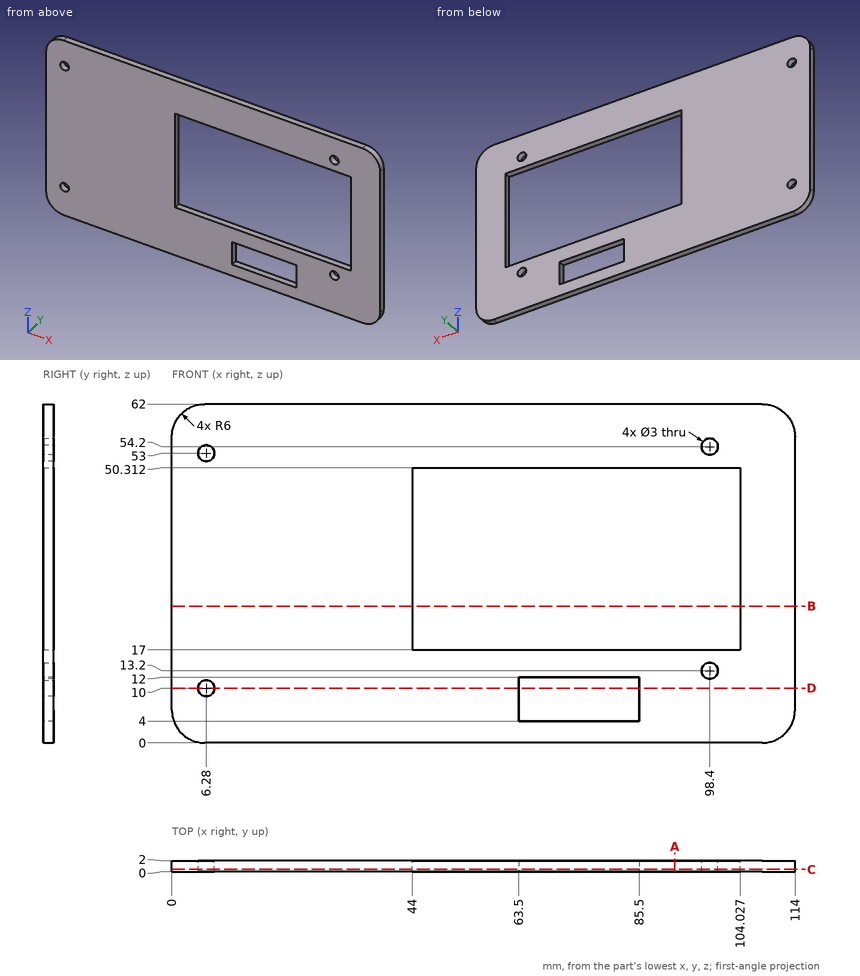
Geometry check sheet. Reference: drawing and pictorial views, mm from the part's lowest x, y, z. Round coordinates to 2 decimals unless told otherwise and drop trailing zeros. Loops run counter-clockwise (first coordinate to the right, second up) from the corner with the lowest first, then second, coordinate; pieces in that order, holes last. Notation, with made-up numbers: M 13,11 L 51,11 A19 cw 51,24 Z; hole C 28.25,-22 d5. An arc over 180 degrees is marked long. One line per item, written item: value.
(1) Sectioned sample at B-B, the plane z = 25. Record the cut outline in (x, y), then the cut area to 3 significant figures.
Computed values:
outline: M 0,0 L 44,0 L 44,2 L 0,2 Z; M 104.03,0 L 114,0 L 114,2 L 104.03,2 Z
area: 108 mm^2
(2) Sectioned sample at C-C, the plane y = 0.45. Record the cut outline in (x, z), then the cut area to 3 significant figures.
Computed values:
outline: M 0,6 A6 ccw 6,0 L 108,0 A6 ccw 114,6 L 114,56 A6 ccw 108,62 L 6,62 A6 ccw 0,56 Z; hole C 6.28,10 d3; hole C 6.28,53 d3; hole M 44,17 L 104.03,17 L 104.03,50.31 L 44,50.31 Z; hole M 63.5,4 L 85.5,4 L 85.5,12 L 63.5,12 Z; hole C 98.4,13.2 d3; hole C 98.4,54.2 d3
area: 4,830 mm^2
(3) Thickness scan on line 1 (Z direction, x = 66, y = 0.1); line 2 (X direction, y = 1.3, z = 10); line 3 (Z direction, x = 98.4, y = 0.6). Record the ranges inside material, lowest first.
Computed values:
line 1: z = 0 to 4, 12 to 17, 50.31 to 62
line 2: x = 0 to 4.78, 7.78 to 63.5, 85.5 to 114
line 3: z = 0 to 11.7, 14.7 to 17, 50.31 to 52.7, 55.7 to 62
(4) Sectioned sample at D-D, the plane z = 10. Record the cut outline in (x, y).
Computed values:
outline: M 0,0 L 4.78,0 L 4.78,2 L 0,2 Z; M 7.78,0 L 63.5,0 L 63.5,2 L 7.78,2 Z; M 85.5,0 L 114,0 L 114,2 L 85.5,2 Z
(5) Depth check by flat-ended pin: pin 1 Ø2.5 at (x, z) = (6.28, 53) entering from -Y. Enter the tip coordinate at first touch or a pass-through.
Computed values:
pin 1: passes through
(6) Sectioned sample at A-A, the plane x = 92. Record the cut outline in (y, z).
Computed values:
outline: M 0,0 L 2,0 L 2,17 L 0,17 Z; M 0,50.31 L 2,50.31 L 2,62 L 0,62 Z
